```python
from build123d import *

# Parameters (mm, degrees)
BOSS_EXTRUDE5_DEPTH   = 12
BOSS_EXTRUDE5_2_DEPTH = 12
BOSS_EXTRUDE6_DEPTH   = 32


with BuildPart() as part:
    # Sketch6 → Boss-Extrude5 (new body)
    with BuildSketch(Plane(origin=(0, 0, 0), x_dir=(1, 0, 0), z_dir=(0, 1, 0))):
        Polygon((-26.75977594, 29.975997565), (-52.75977594, 29.975997565), (-52.75977594, 12.642664232), (-42.75977594, 12.642664232), (-42.75977594, -4.690669102), (-52.75977594, -4.690669102), (-52.75977594, -22.024002435), (-26.75977594, -22.024002435), (-26.75977594, -8.024002435), (-21.75977594, -8.024002435), (-21.75977594, 15.975997565), (-26.75977594, 15.975997565), align=None)
    extrude(amount=BOSS_EXTRUDE5_DEPTH)



with BuildPart() as body_2:
    # Sketch6 → Boss-Extrude5 2 (new body)
    with BuildSketch(Plane(origin=(0, 0, 0), x_dir=(1, 0, 0), z_dir=(0, 1, 0))):
        Polygon((25.24022406, 29.975997565), (-0.75977594, 29.975997565), (-0.75977594, 15.975997565), (-5.75977594, 15.975997565), (-5.75977594, -8.024002435), (-0.75977594, -8.024002435), (-0.75977594, -22.024002435), (25.24022406, -22.024002435), align=None)
    extrude(amount=BOSS_EXTRUDE5_2_DEPTH)


with BuildPart() as part_1:
    add(part.part)

    add(body_2.part)  # Boss-Extrude6 merges body 2
    # Sketch6<3> → Boss-Extrude6 (add)
    with BuildSketch(Plane(origin=(0, 0, 0), x_dir=(1, 0, 0), z_dir=(0, 1, 0))):
        Polygon((-0.75977594, 29.975997565), (-26.75977594, 29.975997565), (-26.75977594, 15.975997565), (-21.75977594, 15.975997565), (-21.75977594, -8.024002435), (-26.75977594, -8.024002435), (-26.75977594, -22.024002435), (-0.75977594, -22.024002435), (-0.75977594, -8.024002435), (-5.75977594, -8.024002435), (-5.75977594, 15.975997565), (-0.75977594, 15.975997565), align=None)
    extrude(amount=BOSS_EXTRUDE6_DEPTH)


solid = part_1.part
```
Can you work these out from the model? Positions are in its coordinate system, mm. A direction names the side the tool comes from. Coordinates: 2 decimals unless noted, no trailing zeros. Write each loop counter-clockwise with the first axis right and the second up, starting at its lowest first coordinate (ties: lowest second). Pieces come first, ordered by that corner, then holes. Notation, with made-up numbers: M -12,-16.5 L 16,-16.5 A27 ccw 16,8.5 Z; hole C 49,-26 d6. An arc over 180 degrees is marked long. Write item = value, one per line. Start each with the question number.
Q1. If we section it at B-B, the plane y = 24.5: Write out the boundary of the cut face in (x, z), then the cut area to 3 significant figures.
Q2. If we section it at D-D, the plane x = -25.5: Write out the boundary of the cut face in (y, z), then the cut area to 3 significant figures.
Q3. On a 3-axis mill with a long thin cutter (end or side, diameter ignored), from which of +Z, -Z, +X, -X, +Y, -Y can I reach the whole of each face in a straight line? I mean faces 5 (the face through (-5.76, 22, -4)), 6 (the face through (-0.76, 22, -23)), 7 (the face through (-48, 6, 4.691)), 8 (the face through (-26.76, 22, -23)). Say none if no direction works.
Q4. If we section it at C-C, the plane z = 11: Write out the boundary of the cut face in (x, y).
Q5. If I drill on L1, parallel to Z at x = -25, y = 24.5; L2, parallel to Y at x = 6.5, z = 20.5; L3, parallel to X at y = 24, z = -12, over which ranges is the centre line in solid material (lowest first)? Write a range as [from, to].
Q6. If we section it at A-A, the plane x = -45: Write out the boundary of the cut face in (y, z), then the cut area to 3 significant figures.
Q7. I'm going to push flat-ended pins straight in: pin 1 (9.5 mm diameter, centred on y = 6, z = 0, fed in from -X); pin 2 (7 mm diameter, centred on y = 23, z = -23, fed in from +X); pin 3 (1.5 mm diameter, centred on x = -28, z = -3, fed in from +Y); pin 4 (15.5 mm diameter, centred on y = 21, z = 16.5, fed in from -X). Where does each tip first touch, or does it pass through?
Q8. Thinking about a two-plate mould opening in Z: for faces 1 (the face through (-48, 6, -12.643)), 2 (the face through (-52.76, 6, 13)), 3 (the face through (-13, 12, -29.976)), 4 (the face through (-24, 22, -15.976)), which applies, released by +Z, released by -Z, zero draft, split by the parting line, or undercut?
Check sheet entries:
q1.outline = M -26.76,-29.98 L -0.76,-29.98 L -0.76,-15.98 L -5.76,-15.98 L -5.76,8.02 L -0.76,8.02 L -0.76,22.02 L -26.76,22.02 L -26.76,8.02 L -21.76,8.02 L -21.76,-15.98 L -26.76,-15.98 Z
q1.area = 1,110 mm²
q2.outline = M 0,-29.98 L 32,-29.98 L 32,-15.98 L 12,-15.98 L 12,8.02 L 32,8.02 L 32,22.02 L 0,22.02 Z
q2.area = 1,180 mm²
q3.face_5 = +X, +Y
q3.face_6 = +Z, -Z, +X, +Y
q3.face_7 = -X, +Y, -Y
q3.face_8 = +Z, -Z, -X, +Y
q4.outline = M -52.76,0 L 25.24,0 L 25.24,12 L -0.76,12 L -0.76,32 L -26.76,32 L -26.76,12 L -52.76,12 Z
q5.L1 = [-29.98, -15.98], [8.02, 22.02]
q5.L2 = [0, 12]
q5.L3 = [-21.76, -5.76]
q6.outline = M 0,-29.98 L 12,-29.98 L 12,-12.64 L 0,-12.64 Z; M 0,4.69 L 12,4.69 L 12,22.02 L 0,22.02 Z
q6.area = 416 mm²
q7.pin_1 = -52.76
q7.pin_2 = -0.76
q7.pin_3 = 12
q7.pin_4 = -26.76
q8.face_1 = undercut
q8.face_2 = zero draft
q8.face_3 = released by -Z
q8.face_4 = undercut
